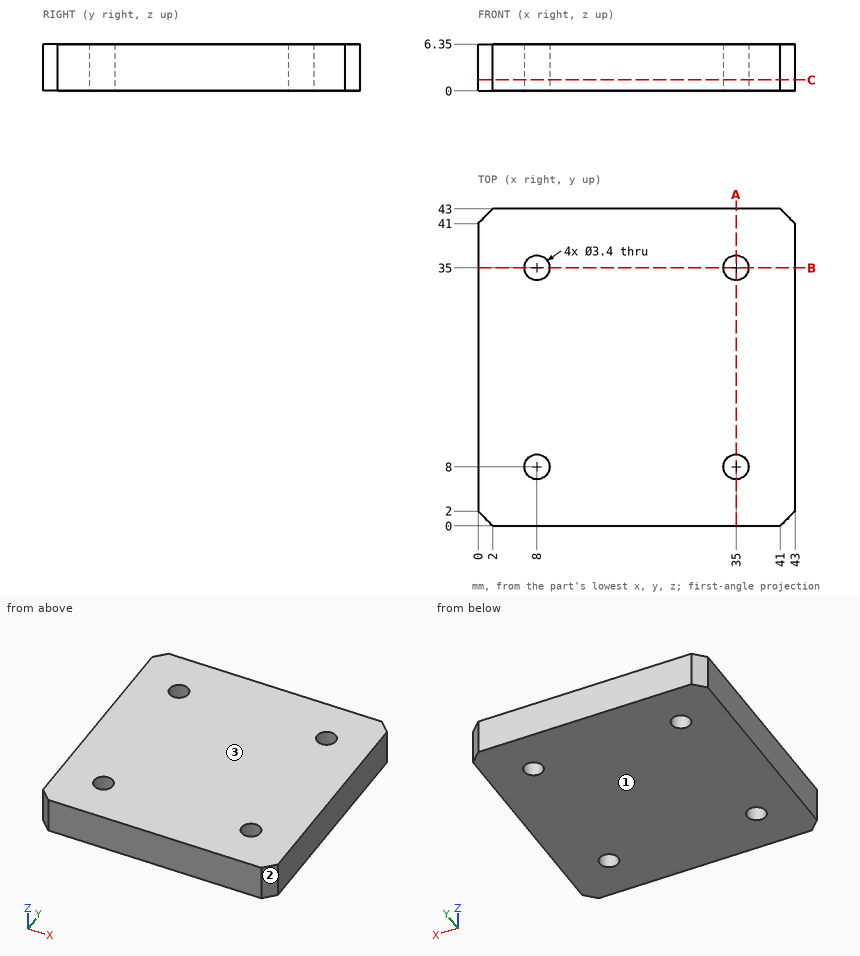
Input: dimensioned drawing with shaded views. Units: mm. Origin: part minimum x, y, z. Give positions to 0.01 mm unless a question says otherwise; leave off trailing zeros. Write each loop counter-clockwise with the first axis right and the second up, starting at its lowest first coordinate (ties: lowest second). Pieces come first, ordered by that corner, then holes.
1. Material intervals for line 1 along Y through (x, z) = (35, 3); line 2 along Y through (x, z) = (7.5, 6), sorted ascending.
2. Section query C-C (z = 1.5). Return the cut outline in (x, y).
3. Pull-direction query (Z, two-part tool) for the marked faces 1, 2 and 3; classes: +Z half, -Z half, draft (parallel to the pull), parting line (faces both ways), or undercut.
4. Section query A-A (x = 35). Return the cut outline in (y, z).
Output values:
1. line 1: y = 0 to 6.3, 9.7 to 33.3, 36.7 to 43
1. line 2: y = 0 to 6.38, 9.62 to 33.38, 36.62 to 43
2. outline: (0, 2) - (2, 0) - (41, 0) - (43, 2) - (43, 41) - (41, 43) - (2, 43) - (0, 41) - close; hole circle Ø3.4 at (8, 8); hole circle Ø3.4 at (8, 35); hole circle Ø3.4 at (35, 8); hole circle Ø3.4 at (35, 35)
3. face 1: -Z half
3. face 2: draft
3. face 3: +Z half
4. outline: (0, 0) - (6.3, 0) - (6.3, 6.35) - (0, 6.35) - close; (9.7, 0) - (33.3, 0) - (33.3, 6.35) - (9.7, 6.35) - close; (36.7, 0) - (43, 0) - (43, 6.35) - (36.7, 6.35) - close
